Verification items for the finished model (mm, model axes). A direction names the side the tool comes from. Give positions to 0.01 mm unless a question says otherwise; leave off trailing zeros. Loops run counter-clockwise (first coordinate to the right, second up) from the corner with the lowest first, then second, coordinate; pieces in that order, holes last. Notation, with made-up numbers: (-20.5, 52) - (26.5, 52) arc R26 cw to (26.5, 71) - close; hole circle Ø10 at (32.5, 6.25). An arc over 180 degrees is marked (long way). Use one line per item in the form item = value.
```python
from build123d import *

# Parameters (mm, degrees)
F0_R       = 32.5
F0_R_2     = 25
F1_DEPTH   = 50
F4_D       = 14
F4_ON_F3_D = 14
F5_R       = 5
F6_R       = 35
F6_R_2     = 25
F7_DEPTH   = 50
F8_R       = 35
F8_R_2     = 25
F9_DEPTH   = 5
F10_DEPTH  = 60
F11_R      = 4.99999


# Not quite as in the source:
# - a fillet or chamfer is up to 0.001 mm smaller than in the source, because OpenCascade refuses the exact size


with BuildPart() as f1:
    # F0 (on Front) → F1 (new body)
    with BuildSketch(Plane.XZ):
        with BuildLine():
            ThreePointArc((-50, 0), (0, -50), (50, 0))
            ThreePointArc((50, 0), (0, 50), (-50, 0))
        make_face()
        Circle(F0_R, mode=Mode.SUBTRACT)
        with BuildLine():
            Line((50, -50), (50, 0))
            ThreePointArc((50, 0), (0, -50), (-50, 0))
            Line((-50, 0), (-50, -50))
            Line((-50, -50), (-110, -50))
            Line((-110, -50), (-110, -75))
            Line((-110, -75), (110, -75))
            Line((110, -75), (110, -50))
            Line((110, -50), (50, -50))
        make_face()
        Circle(F0_R)
        Circle(F0_R_2, mode=Mode.SUBTRACT)
    extrude(amount=F1_DEPTH)

    # F4 (through all)
    with Locations(Plane.XY.offset(-50)):
        with Locations((-80, -25)):
            Hole(F4_D / 2)

    # F4 on F3 (through all)
    with Locations(Plane.XY.offset(-50)):
        with Locations((80, -25)):
            Hole(F4_ON_F3_D / 2)

    # F5
    f5_edges = [f1.edges().sort_by_distance(p)[0] for p in [
        (50, -25, -50),
        (-50, -25, -50),
        (110, -25, -50),
        (-110, -25, -50),
    ]]
    fillet(f5_edges, radius=F5_R)

    # F6 (on face) → F7 (join)
    with BuildSketch(Plane(origin=(0, 0, 0), x_dir=(-1, 0, 0), z_dir=(0, 1, 0))):
        Circle(F6_R)
        Circle(F6_R_2, mode=Mode.SUBTRACT)
    extrude(amount=-F7_DEPTH)

    # F8 (on face) → F9 (join)
    with BuildSketch(Plane.XZ.offset(50)):
        Circle(F8_R)
        Circle(F8_R_2, mode=Mode.SUBTRACT)
    extrude(amount=F9_DEPTH)

    # F10 (add): a face of the model
    f10_faces = [f1.faces().sort_by_distance(p)[0] for p in [
        (-34.0100505063, -55, 0),
    ]]
    extrude(f10_faces, amount=-F10_DEPTH)

    # F11 (radius 5 in the source; OpenCascade refuses exactly that, so slightly less here)
    f11_edges = [f1.edges().sort_by_distance(p)[0] for p in [
        (-35, -50, 0),
        (-35, 0, 0),
    ]]
    fillet(f11_edges, radius=F11_R)


solid = f1.part
```
1. Section check C-C, the plane y = -39. Record the cut outline in (x, z).
Result set:
outline = (-110, -75) - (110, -75) - (110, -55) arc R5 ccw to (105, -50) - (55, -50) arc R5 cw to (50, -45) - (50, 0) arc R50 ccw to (-50, 0) - (-50, -45) arc R5 cw to (-55, -50) - (-105, -50) arc R5 ccw to (-110, -55) - close; hole circle Ø50 at (0, 0)
2. Scan lines: probe 1 along Z at (x, y) = (0, -20.5); probe 2 along Y at (x, z) = (80, -59.75); probe 3 along X at (y, z) = (-16.5, 0). Record each from-to range of solid material in increasing order.
Result set:
probe_1 = -75 to -25, 25 to 50
probe_2 = -50 to -32, -18 to 0
probe_3 = -50 to -25, 25 to 50
3. Tool access check on faces 4 (the flat face through (-50, -25, -22)), 5 (the flat face through (86, -19, -50)), 6 (the cylindrical face through (1.099, -24.65, 49.988)). Record the directions out of +Z, -Z, +X, -X, +Y, -Y that give a thin tool (end or side, any length) a straight path to the whole face; none if there is none.
Result set:
face_4 = +Z, -X, +Y, -Y
face_5 = +Z, +X, +Y, -Y
face_6 = +Z, +Y, -Y
4. Section check A-A, the plane y = -25. Record the cut outline in (x, z), then the cut area to 3 significant figures.
Result set:
outline = (-110, -75) - (-87, -75) - (-87, -50) - (-105, -50) arc R5 ccw to (-110, -55) - close; (-73, -75) - (73, -75) - (73, -50) - (55, -50) arc R5 cw to (50, -45) - (50, 0) arc R50 ccw to (-50, 0) - (-50, -45) arc R5 cw to (-55, -50) - (-73, -50) - close; (87, -75) - (110, -75) - (110, -55) arc R5 ccw to (105, -50) - (87, -50) - close; hole circle Ø50 at (0, 0)
area = 11,800 mm²
5. Section check B-B, the plane x = 80. Record the cut outline in (y, z), then the cut area to 3 significant figures.
Result set:
outline = (-50, -75) - (-32, -75) - (-32, -50) - (-50, -50) - close; (-18, -75) - (0, -75) - (0, -50) - (-18, -50) - close
area = 900 mm²
6. Depth check by flat-ended pin: pin 1 Ø8 at (y, z) = (-43.5, -35.5) entering from -X; pin 2 Ø5 at (x, y) = (-73, -39.5) entering from +Z; pin 3 Ø1.5 at (x, z) = (-80, -60) entering from -Y. Enter the tip coordinate at first touch or a pass-through.
Result set:
pin_1 = -50
pin_2 = -50
pin_3 = -50
7. Draft check along Y on faces 1 (the cylindrical face through (-51, -25, -48)), 2 (the flat face through (-24, -55, 8)), 3 (the cylindrical face through (85.555, -29.259, -62.675)). Enter one of: released by +Y, released by -Y, zero draft, split by the parting line, or undercut.
Result set:
face_1 = zero draft
face_2 = released by -Y
face_3 = undercut
